from build123d import *

# Parameters (mm, degrees)
F1_DEPTH = 19.05
F2_W     = 584.2
F2_H     = 304.8
F2_W_2   = 279.4
F3_DEPTH = 438.15
F5_DEPTH = 19.05
F6_W     = 374.65
F6_H     = 19.05
F7_DEPTH = 609.6


with BuildPart() as f1:
    # F0 (on Front) → F1 (new body)
    with BuildSketch(Plane.XZ):
        Polygon((0, 1320.8), (0, 0), (1219.2, 0), (1219.2, 330.2), (914.4, 330.2), (914.4, 660.4), (609.6, 660.4), (609.6, 990.6), (304.8, 990.6), (304.8, 1320.8), align=None)
    extrude(amount=F1_DEPTH)

    # F2 (on face) → F3 (join)
    with BuildSketch(Plane.XZ.offset(19.05)):
        Polygon((1193.8, 0), (1219.2, 0), (1219.2, 330.2), (914.4, 330.2), (914.4, 660.4), (609.6, 660.4), (609.6, 990.6), (304.8, 990.6), (304.8, 1320.8), (0, 1320.8), (0, 0), (25.4, 0), (25.4, 1295.4), (279.4, 1295.4), (279.4, 0), (304.8, 0), (304.8, 304.8), (889, 304.8), (889, 0), (914.4, 0), (914.4, 304.8), (1193.8, 304.8), align=None)
        with Locations((596.9, 482.6)):
            Rectangle(F2_W, F2_H, mode=Mode.SUBTRACT)
        with Locations((444.5, 812.8)):
            Rectangle(F2_W_2, F2_H, mode=Mode.SUBTRACT)
    extrude(amount=F3_DEPTH)

    # F4 (on face) → F5 (join)
    with BuildSketch(Plane.XZ.offset(457.2)):
        Polygon((609.6, 990.6), (609.6, 1625.6), (0, 1625.6), (0, 1320.8), (304.8, 1320.8), (304.8, 990.6), align=None)
    extrude(amount=-F5_DEPTH)

    # F6 (on face) → F7 (join, through all)
    with BuildSketch(Plane(origin=(0, 0, 0), x_dir=(0, -1, 0), z_dir=(-1, 0, 0))):
        with Locations((625.475, 1616.075)):
            Rectangle(F6_W, F6_H)
    extrude(amount=-F7_DEPTH)


solid = f1.part
For this review, take the finished solid that the model builds, in its own axes (mm). A direction names the side the tool comes from. Coordinates: 2 decimals unless noted, no trailing zeros. Order: outer loops, then holes, each group sorted by start corner. A loop starts at its lowest first (then second) coordinate and runs counter-clockwise, first axis right, second up. Notation, with made-up numbers: (55.25, 56) -> (67.25, 56) arc R13 ccw to (67.25, 64) -> close; hole circle Ø7 at (7.5, 78.5). An arc over 180 degrees is marked (long way). Return JSON: item names as keys, results as strings.
1. The part is to be moulded in two halves that separate along Z. For faces 1 (the flat face through (1052, -235, 304.8)), 2 (the flat face through (1069, -225, 330.2)), 3 (the flat face through (609.6, -258, 855)), 4 (the flat face through (889, -235, 480)), say which applies: +Z half, -Z half, draft (parallel to the pull), parting line (faces both ways), or undercut.
Answer block:
{"face 1": "-Z half", "face 2": "+Z half", "face 3": "draft", "face 4": "undercut"}
2. We need section A-A on x = 133. Write out the cut boundary in (y, z), and give its area (3 significant figures).
Answer block:
{"outline": "(-812.8, 1606.55) -> (-457.2, 1606.55) -> (-457.2, 1295.4) -> (-19.05, 1295.4) -> (-19.05, 0) -> (0, 0) -> (0, 1320.8) -> (-438.15, 1320.8) -> (-438.15, 1625.6) -> (-812.8, 1625.6) -> close", "area": "48,900 mm²"}
3. For line 1 (Z direction, x = 537, y = -435.5); line 2 (X direction, y = -379, z = 401.5); line 3 (Z direction, x = 591.5, y = -408), list the stretches that pass through material, from the lowest coordinate up. Write a range as from..to.
Answer block:
{"line 1": "304.8..330.2, 635..660.4, 965.2..990.6", "line 2": "0..25.4, 279.4..304.8, 889..914.4", "line 3": "304.8..330.2, 635..990.6"}
4. We need section B-B on z = 815. Write out the cut boundary in (x, y).
Answer block:
{"outline": "(0, -457.2) -> (25.4, -457.2) -> (25.4, -19.05) -> (279.4, -19.05) -> (279.4, -457.2) -> (304.8, -457.2) -> (304.8, -19.05) -> (584.2, -19.05) -> (584.2, -457.2) -> (609.6, -457.2) -> (609.6, 0) -> (0, 0) -> close"}
5. For pin 1 Ø1 at (x, z) = (285.5, 372.5) entering from -Y; pin 2 Ø1 at (x, y) = (632.5, -428) entering from -Z; pin 3 Ø12 at (x, z) = (574.5, 435.5) entering from -Y, all flat-tipped, find the tip position at first contact; note any pin that passes through.
Answer block:
{"pin 1": "y = -457.2", "pin 2": "z = 304.8", "pin 3": "y = -19.05"}
6. We need section D-D on x = 528.5. Write out the cut boundary in (y, z).
Answer block:
{"outline": "(-812.8, 1606.55) -> (-457.2, 1606.55) -> (-457.2, 965.2) -> (-19.05, 965.2) -> (-19.05, 660.4) -> (-457.2, 660.4) -> (-457.2, 635) -> (-19.05, 635) -> (-19.05, 330.2) -> (-457.2, 330.2) -> (-457.2, 304.8) -> (-19.05, 304.8) -> (-19.05, 0) -> (0, 0) -> (0, 990.6) -> (-438.15, 990.6) -> (-438.15, 1625.6) -> (-812.8, 1625.6) -> close"}
7. We need section C-C on y = -269.5. State how many separate pieces and enclosed holes the cut face has, and give its area (3 significant figures).
Answer block:
{"separate pieces": "1", "enclosed holes": "2", "area": "151,000 mm²"}
8. Machinability: for faces 5 (the flat face through (301, -633, 1606.55)), 6 (the flat face through (584.2, -235, 811)), 7 (the flat face through (151, -19.05, 657)), which of the approach directions +Z, -Z, +X, -X, +Y, -Y give a long, thin tool a straight path to every point of the face, cutting with its end or side? Answer none if there is none.
Answer block:
{"face 5": "-Z, +X, -X, -Y", "face 6": "-Y", "face 7": "-Z, -Y"}
